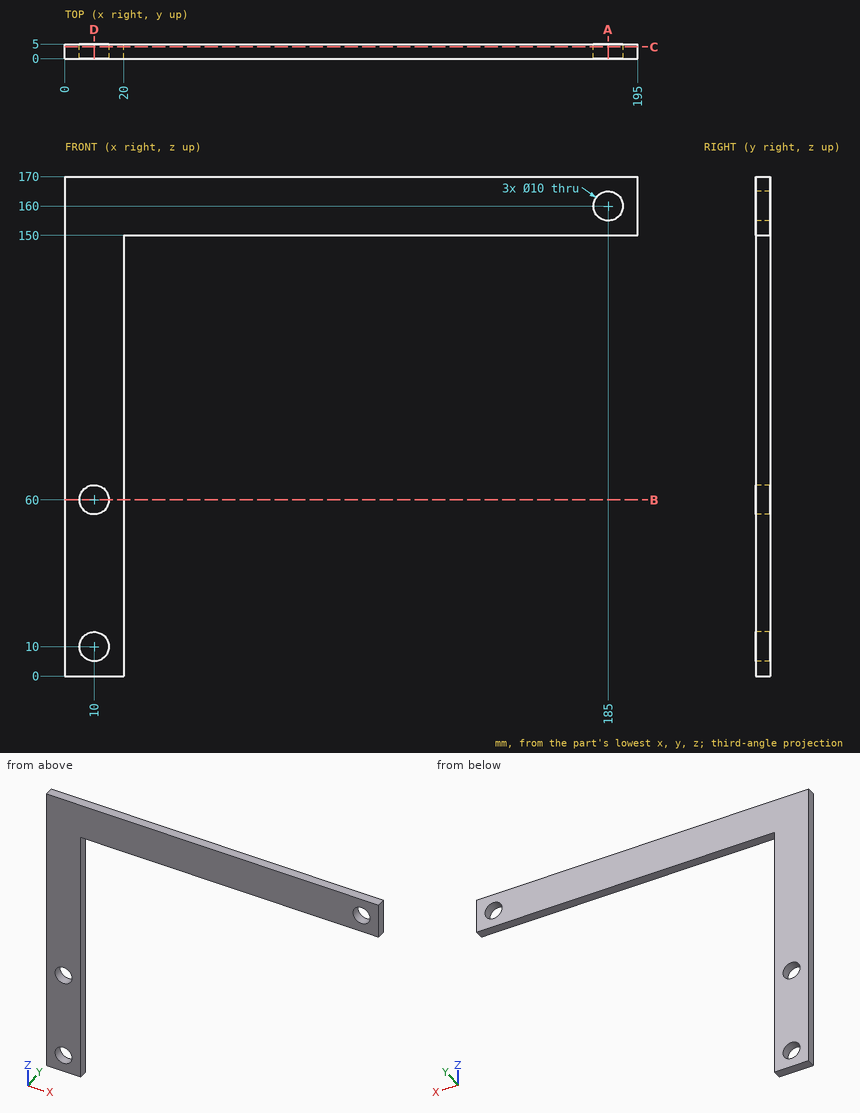
The drawing under review shows one solid part. Ordinate dimensions are in mm from its lowest x, y, z. Round coordinates to 2 decimals unless told otherwise and drop trailing zeros. Loops run counter-clockwise (first coordinate to the right, second up) from the corner with the lowest first, then second, coordinate; pieces in that order, holes last. Notation, with made-up numbers: (43, 82) - (78, 82) arc R14 cw to (78, 103) - close; hole circle Ø5 at (1.5, -17). An arc over 180 degrees is marked (long way). Put each result on its own line as item: value. Start each with the question number.
1. Consider section B-B on z = 60. State the section outline as (x, y) points.
2. Insertion check: P1, Ø3, axis at x = 44.5, y = 3, coming from the -Z side. The pin has a flat end and moves straight along its axis. Give the tip position at first contact, or say it passes through.
3. Consider section A-A on x = 185. State the section outline as (y, z) points.
4. Consider section D-D on x = 10. State the section outline as (y, z) points.
5. Consider section C-C on y = 4.05. State the section outline as (x, z) points.
6. For probe 1 along Z at (x, y) = (10, 1.15); probe 2 along Z at (x, y) = (185, 3.9); probe 3 along Z at (x, y) = (129, 0.85), list the stretches that pass through material, from the lowest coordinate up. Write a range as [from, to].
Result sheet:
1. outline: (0, 0) - (5, 0) - (5, 5) - (0, 5) - close; (15, 0) - (20, 0) - (20, 5) - (15, 5) - close
2. P1: z = 150
3. outline: (0, 150) - (5, 150) - (5, 155) - (0, 155) - close; (0, 165) - (5, 165) - (5, 170) - (0, 170) - close
4. outline: (0, 0) - (5, 0) - (5, 5) - (0, 5) - close; (0, 15) - (5, 15) - (5, 55) - (0, 55) - close; (0, 65) - (5, 65) - (5, 170) - (0, 170) - close
5. outline: (0, 0) - (20, 0) - (20, 150) - (195, 150) - (195, 170) - (0, 170) - close; hole circle Ø10 at (10, 10); hole circle Ø10 at (10, 60); hole circle Ø10 at (185, 160)
6. probe 1: [0, 5], [15, 55], [65, 170]
6. probe 2: [150, 155], [165, 170]
6. probe 3: [150, 170]
